```python
from build123d import *

# Parameters (mm, degrees)
BOSS_EXTRUDE1_DEPTH = 2.4
CUT_EXTRUDE1_REACH  = 98.968
SKETCH4_W           = 13
SKETCH4_H           = 8
SKETCH4_W_2         = 90
SKETCH4_H_2         = 71
SKETCH4_R           = 3
CUT_EXTRUDE2_DEPTH  = 0.45
CUT_EXTRUDE3_REACH  = 98.958
FILLET1_R           = 5


with BuildPart() as part:
    # Sketch1 → Boss-Extrude1 (new body)
    with BuildSketch(Plane.XY):
        with BuildLine():
            Line((66, 0), (-5, 71))
            Line((-5, 71), (-7, 71))
            Line((-7, 71), (-7, 69.414213562))
            ThreePointArc((-7, 69.414213562), (-7, 68), (-8.414213562, 68))
            Line((-8.414213562, 68), (-25.585786438, 68))
            ThreePointArc((-25.585786438, 68), (-27, 68), (-27, 69.414213562))
            Line((-27, 69.414213562), (-27, 71))
            Line((-27, 71), (-29, 71))
            Line((-29, 71), (-34, 66))
            Line((-34, 66), (-66, 66))
            Line((-66, 66), (-66, -66))
            Line((-66, -66), (-47.414213562, -66))
            ThreePointArc((-47.414213562, -66), (-46, -66), (-46, -67.414213562))
            Line((-46, -67.414213562), (-46, -69))
            Line((-46, -69), (-40, -69))
            Line((-40, -69), (-40, -67.414213562))
            ThreePointArc((-40, -67.414213562), (-40, -66), (-38.585786438, -66))
            Line((-38.585786438, -66), (38.585786438, -66))
            ThreePointArc((38.585786438, -66), (40, -66), (40, -67.414213562))
            Line((40, -67.414213562), (40, -69))
            Line((40, -69), (46, -69))
            Line((46, -69), (46, -67.414213562))
            ThreePointArc((46, -67.414213562), (46, -66), (47.414213562, -66))
            Line((47.414213562, -66), (66, -66))
            Line((66, -66), (66, 0))
        make_face()
    extrude(amount=BOSS_EXTRUDE1_DEPTH)

    # Sketch3 → Cut-Extrude1 (cut, up to next)
    with BuildSketch(Plane.XY.offset(2.4), mode=Mode.PRIVATE) as cut_extrude1_sk1:
        with BuildLine():
            Line((-60.75, -58), (-60.75, -55))
            ThreePointArc((-60.75, -55), (-61.75, -54), (-62.75, -55))
            Line((-62.75, -55), (-62.75, -58))
            ThreePointArc((-62.75, -58), (-61.75, -59), (-60.75, -58))
        make_face()
    cut_extrude1_tool1 = extrude(cut_extrude1_sk1.sketch, amount=-CUT_EXTRUDE1_REACH, mode=Mode.PRIVATE) & part.part
    # Sketch3 → Cut-Extrude1 (cut, up to next)
    with BuildSketch(Plane.XY.offset(2.4), mode=Mode.PRIVATE) as cut_extrude1_sk2:
        with BuildLine():
            ThreePointArc((-55.25, -55), (-56.25, -54), (-57.25, -55))
            Line((-57.25, -55), (-57.25, -58))
            ThreePointArc((-57.25, -58), (-56.25, -59), (-55.25, -58))
            Line((-55.25, -58), (-55.25, -55))
        make_face()
    cut_extrude1_tool2 = extrude(cut_extrude1_sk2.sketch, amount=-CUT_EXTRUDE1_REACH, mode=Mode.PRIVATE) & part.part
    # Sketch3 → Cut-Extrude1 (cut, up to next)
    with BuildSketch(Plane.XY.offset(2.4), mode=Mode.PRIVATE) as cut_extrude1_sk3:
        with BuildLine():
            ThreePointArc((-55.25, -40), (-56.25, -39), (-57.25, -40))
            Line((-57.25, -40), (-57.25, -43))
            ThreePointArc((-57.25, -43), (-56.25, -44), (-55.25, -43))
            Line((-55.25, -43), (-55.25, -40))
        make_face()
    cut_extrude1_tool3 = extrude(cut_extrude1_sk3.sketch, amount=-CUT_EXTRUDE1_REACH, mode=Mode.PRIVATE) & part.part
    # Sketch3 → Cut-Extrude1 (cut, up to next)
    with BuildSketch(Plane.XY.offset(2.4), mode=Mode.PRIVATE) as cut_extrude1_sk4:
        with BuildLine():
            Line((-60.75, -43), (-60.75, -40))
            ThreePointArc((-60.75, -40), (-61.75, -39), (-62.75, -40))
            Line((-62.75, -40), (-62.75, -43))
            ThreePointArc((-62.75, -43), (-61.75, -44), (-60.75, -43))
        make_face()
    cut_extrude1_tool4 = extrude(cut_extrude1_sk4.sketch, amount=-CUT_EXTRUDE1_REACH, mode=Mode.PRIVATE) & part.part
    # Sketch3 → Cut-Extrude1 (cut, up to next)
    with BuildSketch(Plane.XY.offset(2.4), mode=Mode.PRIVATE) as cut_extrude1_sk5:
        with BuildLine():
            Line((-60.75, -28), (-60.75, -25))
            ThreePointArc((-60.75, -25), (-61.75, -24), (-62.75, -25))
            Line((-62.75, -25), (-62.75, -28))
            ThreePointArc((-62.75, -28), (-61.75, -29), (-60.75, -28))
        make_face()
    cut_extrude1_tool5 = extrude(cut_extrude1_sk5.sketch, amount=-CUT_EXTRUDE1_REACH, mode=Mode.PRIVATE) & part.part
    # Sketch3 → Cut-Extrude1 (cut, up to next)
    with BuildSketch(Plane.XY.offset(2.4), mode=Mode.PRIVATE) as cut_extrude1_sk6:
        with BuildLine():
            ThreePointArc((-55.25, -25), (-56.25, -24), (-57.25, -25))
            Line((-57.25, -25), (-57.25, -28))
            ThreePointArc((-57.25, -28), (-56.25, -29), (-55.25, -28))
            Line((-55.25, -28), (-55.25, -25))
        make_face()
    cut_extrude1_tool6 = extrude(cut_extrude1_sk6.sketch, amount=-CUT_EXTRUDE1_REACH, mode=Mode.PRIVATE) & part.part
    # Sketch3 → Cut-Extrude1 (cut, up to next)
    with BuildSketch(Plane.XY.offset(2.4), mode=Mode.PRIVATE) as cut_extrude1_sk7:
        with BuildLine():
            Line((-60.75, -13), (-60.75, -10))
            ThreePointArc((-60.75, -10), (-61.75, -9), (-62.75, -10))
            Line((-62.75, -10), (-62.75, -13))
            ThreePointArc((-62.75, -13), (-61.75, -14), (-60.75, -13))
        make_face()
    cut_extrude1_tool7 = extrude(cut_extrude1_sk7.sketch, amount=-CUT_EXTRUDE1_REACH, mode=Mode.PRIVATE) & part.part
    # Sketch3 → Cut-Extrude1 (cut, up to next)
    with BuildSketch(Plane.XY.offset(2.4), mode=Mode.PRIVATE) as cut_extrude1_sk8:
        with BuildLine():
            ThreePointArc((-55.25, -10), (-56.25, -9), (-57.25, -10))
            Line((-57.25, -10), (-57.25, -13))
            ThreePointArc((-57.25, -13), (-56.25, -14), (-55.25, -13))
            Line((-55.25, -13), (-55.25, -10))
        make_face()
    cut_extrude1_tool8 = extrude(cut_extrude1_sk8.sketch, amount=-CUT_EXTRUDE1_REACH, mode=Mode.PRIVATE) & part.part
    add(cut_extrude1_tool1.solids().sort_by_distance((-61.75, -56.5, 2.4))[0], mode=Mode.SUBTRACT)
    add(cut_extrude1_tool2.solids().sort_by_distance((-56.25, -56.5, 2.4))[0], mode=Mode.SUBTRACT)
    add(cut_extrude1_tool3.solids().sort_by_distance((-56.25, -41.5, 2.4))[0], mode=Mode.SUBTRACT)
    add(cut_extrude1_tool4.solids().sort_by_distance((-61.75, -41.5, 2.4))[0], mode=Mode.SUBTRACT)
    add(cut_extrude1_tool5.solids().sort_by_distance((-61.75, -26.5, 2.4))[0], mode=Mode.SUBTRACT)
    add(cut_extrude1_tool6.solids().sort_by_distance((-56.25, -26.5, 2.4))[0], mode=Mode.SUBTRACT)
    add(cut_extrude1_tool7.solids().sort_by_distance((-61.75, -11.5, 2.4))[0], mode=Mode.SUBTRACT)
    add(cut_extrude1_tool8.solids().sort_by_distance((-56.25, -11.5, 2.4))[0], mode=Mode.SUBTRACT)

    # Sketch4 → Cut-Extrude2 (cut)
    with BuildSketch(Plane.XY.offset(2.4)):
        with Locations((-59.5, -49)):
            Rectangle(SKETCH4_W, SKETCH4_H)
        with Locations((-8, -17.5)):
            Rectangle(SKETCH4_W_2, SKETCH4_H_2)
        with Locations((-50.878679656, 15.878679656)):
            Circle(SKETCH4_R)
        with Locations((34.878679656, 15.878679656)):
            Circle(SKETCH4_R)
        with Locations((34.878679656, -50.878679656)):
            Circle(SKETCH4_R)
    extrude(amount=-CUT_EXTRUDE2_DEPTH, mode=Mode.SUBTRACT)

    # Sketch5 → Cut-Extrude3 (cut, up to next)
    with BuildSketch(Plane.XY.offset(1.95), mode=Mode.PRIVATE) as cut_extrude3_sk1:
        with BuildLine():
            Line((-66, -45), (-54, -45))
            ThreePointArc((-54, -45), (-53.292893219, -45.292893219), (-53, -46))
            Line((-53, -46), (-53, -52))
            ThreePointArc((-53, -52), (-53.292893219, -52.707106781), (-54, -53))
            Line((-54, -53), (-66, -53))
            Line((-66, -53), (-66, -45))
        make_face()
    cut_extrude3_tool1 = extrude(cut_extrude3_sk1.sketch, amount=-CUT_EXTRUDE3_REACH, mode=Mode.PRIVATE) & part.part
    add(cut_extrude3_tool1.solids().sort_by_distance((-59.526011, -49, 1.95))[0], mode=Mode.SUBTRACT)

    # Fillet1
    fillet1_edges = [part.edges().sort_by_distance(p)[0] for p in [
        (-34, 66, 1.2),
        (66, 0, 1.2),
    ]]
    fillet(fillet1_edges, radius=FILLET1_R)


solid = part.part
```
Model file for the job. Use its own axes, mm. A direction names the side the tool comes from. Give positions to 0.01 mm unless a question says otherwise; leave off trailing zeros. Order: outer loops, then holes, each group sorted by start corner. A loop starts at its lowest first (then second) coordinate and runs counter-clockwise, first axis right, second up.
1) 3-axis set-ups, long thin cutter, end or side, ignore diameter. For faces 5 (the flat face through (-1, 33, 2.4)), 6 (the cylindrical face through (37, -53, 2.2)): which of +Z, -Z, +X, -X, +Y, -Y reach the whole face in a straight line?
2) Saw through at C-C, the plane y = -35. Write the cut outline in (x, z).
3) Saw through at B-B, the plane z = 1.25. Count the separate pieces of the cut face and the enclosed holes in it, then the cut area to 3 significant figures.
4) Pin check, flat tips, straight feed: pin 1 (0.8 mm diameter, centred on y = -68, z = 1.5, fed in from -X); pin 2 (0.5 mm diameter, centred on y = 70.5, z = 1, fed in from +X); pin 3 (1 mm diameter, centred on x = -49.5, y = -18, fed in from +Z). Stop position of each tip, or through.
5) Saw through at D-D, the plane y = 55. Write the cut outline in (x, z), then the cut area to 3 significant figures.
6) Saw through at A-A, the plane y = 6.5. Write the cut outline in (x, z), then the cut area to 3 significant figures.
7) Mould opens along X. For faces 1 (the flat face through (30, 36, 1)), 2 (the flat face through (-1, 2, 0)), 3 (the flat face through (-31, 69, 1)), 4 (the cylindrical face through (-53, 18, 2.2)) say: +X half, -X half, draft (parallel to the pull), parting line (faces both ways), or undercut.
8) Wall check: probe 1 along X at (y, z) = (-40, 1.1); probe 2 along Y at (x, z) = (-60, 0.75). Give the ranges that are in metal, low to high.
Computed:
1. face 5: +Z, +X, -X, +Y, -Y
1. face 6: +Z
2. outline: (-66, 0) - (66, 0) - (66, 2.4) - (37, 2.4) - (37, 1.95) - (-53, 1.95) - (-53, 2.4) - (-66, 2.4) - close
3. separate pieces: 1
3. enclosed holes: 8
3. area: 15,200 mm2
4. pin 1: stops at x = -46
4. pin 2: stops at x = -4.25
4. pin 3: stops at z = 1.95
5. outline: (-66, 0) - (11, 0) - (11, 2.4) - (-66, 2.4) - close
5. area: 185 mm2
6. outline: (-66, 0) - (59.5, 0) - (59.5, 2.4) - (37, 2.4) - (37, 1.95) - (-53, 1.95) - (-53, 2.4) - (-66, 2.4) - close
6. area: 261 mm2
7. face 1: +X half
7. face 2: draft
7. face 3: -X half
7. face 4: undercut
8. probe 1: x = -66 to -62.75, -60.75 to -57.25, -55.25 to 66
8. probe 2: y = -66 to -53, -45 to 66
